from build123d import *

# Parameters (mm, degrees)
SKETCH1_R           = 1.2
BOSS_EXTRUDE1_DEPTH = 0.79375
FILLET1_R           = 2


with BuildPart() as part:
    # Sketch1 → Boss-Extrude1 (new body)
    with BuildSketch(Plane(origin=(0, 0, 0), x_dir=(1, 0, 0), z_dir=(0, 1, 0))):
        Polygon((0, 0), (30, 0), (27.816178594, 6), (2.183821406, 6), align=None)
        with Locations(Location((15, 3.4, 0), (0, 0, 270))):
            Circle(SKETCH1_R, mode=Mode.SUBTRACT)
    extrude(amount=BOSS_EXTRUDE1_DEPTH)

    # Fillet1
    fillet1_edges = [part.edges().sort_by_distance(p)[0] for p in [
        (2.183821406, 0.396875, -6),
        (27.816178594, 0.396875, -6),
        (30, 0.396875, 0),
        (0, 0.396875, 0),
    ]]
    fillet(fillet1_edges, radius=FILLET1_R)


solid = part.part
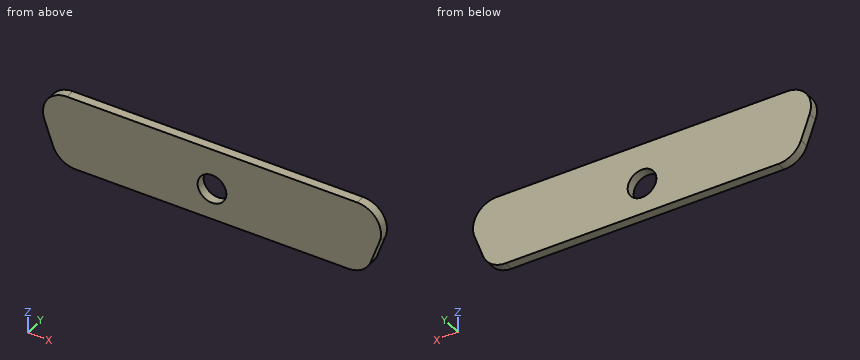
Could you check a few things on this model? Use its own coordinates, in mm. Coordinates: 2 decimals unless noted, no trailing zeros. Order: outer loops, then holes, each group sorted by start corner. A loop starts at its lowest first (then second) coordinate and runs counter-clockwise, first axis right, second up.
Q1. Suppose I cut it at A-A on y = 0.65. Please give me the cut outline in (x, z), and give its area (3 significant figures).
Q2. Suppose I cut it at C-C on z = -3.4. Please give me the cut outline in (x, y), and give its area (3 significant figures).
Q3. Please list where these lines run through material, in increasing order: L1, parallel to X at y = 0.7, z = -4.15; L2, parallel to X at y = 0.35, z = -3.4; L3, parallel to X at y = 0.7, z = -2.15.
Q4. Suppose I cut it at B-B on x = 15. Please give me the cut outline in (y, z), and give its area (3 significant figures).
Q5. Suppose I cut it at D-D on z = -5.55. Please give me the cut outline in (x, y), and give its area (3 significant figures).
Answer:
1. outline: (0.98, -2.68) - (1.7, -4.68) arc R2 ccw to (3.58, -6) - (26.42, -6) arc R2 ccw to (28.3, -4.68) - (29.02, -2.68) arc R2 ccw to (27.14, 0) - (2.86, 0) arc R2 ccw to start; hole circle Ø2.4 at (15, -3.4)
1. area: 158 mm2
2. outline: (1.24, 0) - (13.8, 0) - (13.8, 0.79) - (1.24, 0.79) - close; (16.2, 0) - (28.76, 0) - (28.76, 0.79) - (16.2, 0.79) - close
2. area: 19.9 mm2
3. L1: x = 1.51 to 14.06, 15.94 to 28.49
3. L2: x = 1.24 to 13.8, 16.2 to 28.76
3. L3: x = 0.86 to 29.14
4. outline: (0, -6) - (0.79, -6) - (0.79, -4.6) - (0, -4.6) - close; (0, -2.2) - (0.79, -2.2) - (0.79, 0) - (0, 0) - close
4. area: 2.86 mm2
5. outline: (2.32, 0) - (27.68, 0) - (27.68, 0.79) - (2.32, 0.79) - close
5. area: 20.1 mm2
